The model under review builds one solid part; all positions refer to its coordinate system, in mm. Round coordinates to 2 decimals unless told otherwise and drop trailing zeros. Order: outer loops, then holes, each group sorted by start corner. A loop starts at its lowest first (then second) coordinate and runs counter-clockwise, first axis right, second up.
1) Consider section C-C (y = 1.75). Give the number of separate pieces and of enclosed holes in the cut face, then the cut area to 3 significant figures.
2) Consider section B-B (z = 508). Give the boundary of the cut face in (x, y), then the cut area to 3 significant figures.
3) Consider section A-A (x = 55). Give the boundary of the cut face in (y, z), then the cut area to 3 significant figures.
4) Clearance check with a flat-ended pin moving along its axis: P1, Ø2.5, axis at x = 50.23, z = 604.06, coming from the -Y side. State where the tip first meets the part, or that it passes through.
5) To check wall thickness, follow L1, parallel to Z at x = 67, y = 1.75; L2, parallel to Z at x = 94, y = 1.75; L3, parallel to X at y = 1.5, z = 564. State the ranges of each line that lie inside material, in increasing order.
from build123d import *

# Parameters (mm, degrees)
SKETCH1_W           = 128
SKETCH1_H           = 150.8
SKETCH1_R           = 30
SKETCH1_R_2         = 3.1
BOSS_EXTRUDE1_DEPTH = 6.35
FILLET1_R           = 3
SKETCH3_R           = 1.985
CUT_EXTRUDE1_DEPTH  = 637.633938538


with BuildPart() as part:
    # Sketch1 → Boss-Extrude1 (new body)
    with BuildSketch(Plane(origin=(0, 0, 0), x_dir=(1, 0, 0), z_dir=(0, 1, 0))):
        with Locations((77.127334094, -545.362051651)):
            Rectangle(SKETCH1_W, SKETCH1_H)
        with Locations(Location((76.627334094, -553.262051651, 0), (0, 0, 270))):
            Circle(SKETCH1_R, mode=Mode.SUBTRACT)
        with Locations(Location((25.827334094, -482.662051651, 0), (0, 0, 270))):
            Circle(SKETCH1_R_2, mode=Mode.SUBTRACT)
        with Locations(Location((128.427334094, -482.662051651, 0), (0, 0, 270))):
            Circle(SKETCH1_R_2, mode=Mode.SUBTRACT)
        with Locations(Location((25.827334094, -608.062051651, 0), (0, 0, 270))):
            Circle(SKETCH1_R_2, mode=Mode.SUBTRACT)
        with Locations(Location((25.827334094, -507.862051651, 0), (0, 0, 270))):
            Circle(SKETCH1_R_2, mode=Mode.SUBTRACT)
    extrude(amount=BOSS_EXTRUDE1_DEPTH)

    # Fillet1
    fillet1_edges = [part.edges().sort_by_distance(p)[0] for p in [
        (141.127334094, 3.175, 620.762051651),
        (13.127334094, 3.175, 620.762051651),
        (13.127334094, 3.175, 469.962051651),
        (141.127334094, 3.175, 469.962051651),
    ]]
    fillet(fillet1_edges, radius=FILLET1_R)

    # Sketch3 → Cut-Extrude1 (cut, through all)
    with BuildSketch(Plane(origin=(0, 6.35, 0), x_dir=(1, 0, 0), z_dir=(0, 1, 0))):
        with Locations(Location((25.827334094, -526.868476675, 0), (0, 0, 270))):
            Circle(SKETCH3_R)
        with Locations(Location((103.020909069, -502.462051651, 0), (0, 0, 270))):
            Circle(SKETCH3_R)
        with Locations(Location((127.427334094, -579.655626627, 0), (0, 0, 270))):
            Circle(SKETCH3_R)
        with Locations(Location((50.233759118, -604.062051651, 0), (0, 0, 270))):
            Circle(SKETCH3_R)
    extrude(amount=-CUT_EXTRUDE1_DEPTH, mode=Mode.SUBTRACT)


solid = part.part
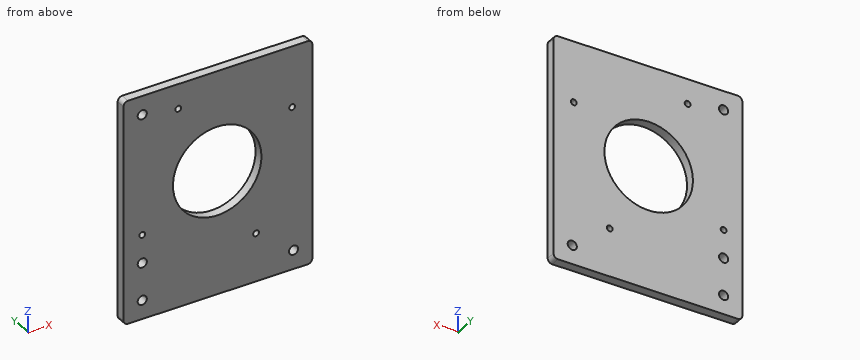
Answer below:
1. separate pieces: 1
1. enclosed holes: 9
1. area: 16,300 mm2
2. outline: (13.13, 0) - (22.73, 0) - (22.73, 6.35) - (13.13, 6.35) - close; (28.92, 0) - (141.13, 0) - (141.13, 6.35) - (28.92, 6.35) - close
2. area: 773 mm2
3. outline: (0, 469.96) - (6.35, 469.96) - (6.35, 532.47) - (0, 532.47) - close; (0, 574.05) - (6.35, 574.05) - (6.35, 620.76) - (0, 620.76) - close
3. area: 694 mm2
4. P1: passes through
5. L1: z = 469.96 to 524.85, 581.68 to 620.76
5. L2: z = 469.96 to 528.8, 577.72 to 620.76
5. L3: x = 13.13 to 48.61, 104.64 to 141.13
